from build123d import *

# Parameters (mm, degrees)
CROQUIS1_R              = 1.5
SALIENTE_EXTRUIR1_DEPTH = 3
CROQUIS2_W              = 20
CROQUIS2_H              = 2
SALIENTE_EXTRUIR2_DEPTH = 2
REDONDEO1_R             = 1


with BuildPart() as part:
    # Croquis1 → Saliente-Extruir1 (new body)
    with BuildSketch(Plane(origin=(0, 0, 0), x_dir=(1, 0, 0), z_dir=(0, 1, 0))):
        Polygon((-15, -5), (15, -5), (15, -8), (25, -8), (25, 8), (15, 8), (15, 5), (-15, 5), (-15, 8), (-25, 8), (-25, -8), (-15, -8), align=None)
        with Locations(Location((0, 0, 0), (0, 0, 270))):
            Circle(CROQUIS1_R, mode=Mode.SUBTRACT)
    extrude(amount=SALIENTE_EXTRUIR1_DEPTH)

    # Croquis2 → Saliente-Extruir2 (add)
    with BuildSketch(Plane(origin=(0, 3, 0), x_dir=(1, 0, 0), z_dir=(0, 1, 0))):
        with Locations((0, 4)):
            Rectangle(CROQUIS2_W, CROQUIS2_H)
        with Locations((0, -4)):
            Rectangle(CROQUIS2_W, CROQUIS2_H)
    extrude(amount=SALIENTE_EXTRUIR2_DEPTH)

    # Redondeo1
    redondeo1_edges = [part.edges().sort_by_distance(p)[0] for p in [
        (-15, 1.5, -8),
        (-15, 1.5, -5),
        (15, 1.5, -5),
        (15, 1.5, -8),
        (25, 1.5, -8),
        (25, 1.5, 8),
        (15, 1.5, 8),
        (15, 1.5, 5),
        (-15, 1.5, 5),
        (-15, 1.5, 8),
        (-25, 1.5, 8),
        (-25, 1.5, -8),
    ]]
    fillet(redondeo1_edges, radius=REDONDEO1_R)


solid = part.part
Geometry check sheet. Reference: the model listing, model coordinates, mm. A direction names the side the tool comes from. Coordinates: 2 decimals unless noted, no trailing zeros. Order: outer loops, then holes, each group sorted by start corner. A loop starts at its lowest first (then second) coordinate and runs counter-clockwise, first axis right, second up. Notation, with made-up numbers: (69, 3) - (78, 3) arc R31 cw to (78, 30) - close; hole circle Ø7 at (12, 71.5). An arc over 180 degrees is marked (long way). Answer in a Markdown table with one row per item. Add a question column.
1) Material ranges on line 1 along X through (y, z) = (2.45, -6.5); line 2 along X through (y, z) = (1.65, 0); line 3 along Z through (x, y) = (4, 0.8), recorded low to high. Write a range as [from, to].
2) Cross-section at B-B, the plane y = 0.9. Record the cut outline in (x, z), then the cut area to 3 significant figures.
3) Cross-section at A-A, the plane x = 0. Record the cut outline in (y, z).
4) Cross-section at D-D, the plane y = 4.5. Record the cut outline in (x, z), then the cut area to 3 significant figures.
5) Cross-section at C-C, the plane z = 6.5. Record the cut outline in (x, y).
6) Set-up check for faces 4 (the cylindrical face through (-15.285, 1.521, 7.699)), 5 (the cylindrical face through (-15.301, 1.521, -7.715)), 6 (the flat face through (-10, 4, 4)): record each of +Z, -Z, +X, -X, +Y, -Y from which the full face is reachable in a straight line by a thin tool's end or side.
7) Release check for a two-part mould opening along X. For faces 1 (the flat face through (0, 5, -4)), 2 (the flat face through (-10, 4, -4)), 3 (the cylindrical face through (14.715, 1.521, -5.301)) record: +X half, -X half, draft (parallel to the pull), parting line (faces both ways), or undercut.
8) Gauge pin test, flat ends, axial feed: P1, Ø2.5, axis at x = 0, z = 0, coming from the +Y side; P2, Ø1.5, axis at x = 5, y = 2, coming from the -Z side; P3, Ø4, axis at x = -13.5, z = 1.5, coming from the +Y side; P4, Ø1, axis at y = 4, z = 4, coming from the +X side. Record the tip position at first contact, or that the pin passes through.
Check result:
| question | item | result |
|---|---|---|
| 1 | line 1 | x = [-25, -15], [15, 25] |
| 1 | line 2 | x = [-25, -1.5], [1.5, 25] |
| 1 | line 3 | z = [-5, 5] |
| 2 | outline | (-25, -7) arc R1 ccw to (-24, -8) - (-16, -8) arc R1 ccw to (-15, -7) - (-15, -6) arc R1 cw to (-14, -5) - (14, -5) arc R1 cw to (15, -6) - (15, -7) arc R1 ccw to (16, -8) - (24, -8) arc R1 ccw to (25, -7) - (25, 7) arc R1 ccw to (24, 8) - (16, 8) arc R1 ccw to (15, 7) - (15, 6) arc R1 cw to (14, 5) - (-14, 5) arc R1 cw to (-15, 6) - (-15, 7) arc R1 ccw to (-16, 8) - (-24, 8) arc R1 ccw to (-25, 7) - close; hole circle Ø3 at (0, 0) |
| 2 | area | 612 mm² |
| 3 | outline | (0, -5) - (5, -5) - (5, -3) - (3, -3) - (3, -1.5) - (0, -1.5) - close; (0, 1.5) - (3, 1.5) - (3, 3) - (5, 3) - (5, 5) - (0, 5) - close |
| 4 | outline | (-10, -5) - (10, -5) - (10, -3) - (-10, -3) - close; (-10, 3) - (10, 3) - (10, 5) - (-10, 5) - close |
| 4 | area | 80.0 mm² |
| 5 | outline | (-25, 0) - (-15, 0) - (-15, 3) - (-25, 3) - close; (15, 0) - (25, 0) - (25, 3) - (15, 3) - close |
| 6 | face 4 | +Z, +Y, -Y |
| 6 | face 5 | -Z, +Y, -Y |
| 6 | face 6 | +Z, -Z, -X, +Y |
| 7 | face 1 | draft |
| 7 | face 2 | -X half |
| 7 | face 3 | undercut |
| 8 | P1 | passes through |
| 8 | P2 | stops at z = -5 |
| 8 | P3 | stops at y = 3 |
| 8 | P4 | stops at x = 10 |
